from build123d import *

# Parameters (mm, degrees)
F2_R     = 0.99999
F3_R     = 2.75
F4_DEPTH = 7.5
F5_R     = 1.75
F6_DEPTH = 9.5
F7_SIZE  = 0.5


# Not quite as in the source:
# - a fillet or chamfer is up to 0.001 mm smaller than in the source, because OpenCascade refuses the exact size


with BuildPart() as f1:
    # F0 (on Front) → F1 (revolve)
    with BuildSketch(Plane.XZ):
        Polygon((0, 4), (0, 0), (17, 0), (17, 3.5), (12, 3.5), (6, 5), (6, 4), align=None)
    revolve(axis=Axis((8.5, 0, 0), (-1, 0, 0)))

    # F2 (radius 1 in the source; OpenCascade refuses exactly that, so slightly less here)
    f2_edges = [f1.edges().sort_by_distance(p)[0] for p in [
        (6, 0, -4),
    ]]
    fillet(f2_edges, radius=F2_R)

    # F3 (on face) → F4 (cut)
    with BuildSketch(Plane.YZ.offset(17)):
        Circle(F3_R)
    extrude(amount=-F4_DEPTH, mode=Mode.SUBTRACT)

    # F5 (on face) → F6 (cut, through all)
    with BuildSketch(Plane(origin=(0, 0, 0), x_dir=(0, -1, 0), z_dir=(-1, 0, 0))):
        Circle(F5_R)
    extrude(amount=-F6_DEPTH, mode=Mode.SUBTRACT)

    # F7
    f7_edges = [f1.edges().sort_by_distance(p)[0] for p in [
        (0, 0, -4),
        (0, 1.75, 0),
    ]]
    chamfer(f7_edges, length=F7_SIZE)


solid = f1.part
Verification items for the finished model (mm, model axes). A direction names the side the tool comes from. Give positions to 0.01 mm unless a question says otherwise; leave off trailing zeros. Loops run counter-clockwise (first coordinate to the right, second up) from the corner with the lowest first, then second, coordinate; pieces in that order, holes last. Notation, with made-up numbers: (-19.5, -31.5) - (34.5, -31.5) arc R8 cw to (34.5, -19.5) - close; hole circle Ø9 at (1, 20). An arc over 180 degrees is marked (long way). Write item = value, one per line. Start each with the question number.
Q1. Tool access check on faces 4 (the face through (4.937, -1.617, -0.67)), 5 (the face through (9.5, 2, 0)), 6 (the face through (2.719, -3.905, -0.867)). Record the directions out of +Z, -Z, +X, -X, +Y, -Y that give a thin tool (end or side, any length) a straight path to the whole face; none if there is none.
Q2. Cross-section at C-C, the plane x = 2. Enter the section's corners in (y, z), and give its area (3 significant figures).
Q3. Cross-section at D-D, the plane x = 7.5. Enter the section's corners in (y, z) (3 decimals).
Q4. Mould release check, pull along Z, two halves, no side actions. Record for faces 1 (the face through (0, -0.7, 2.3)), 2 (the face through (10.291, -3.834, -0.851)), 3 (the face through (13.302, -0.596, -2.685)): released by +Z, released by -Z, zero draft, split by the parting line, or undercut.
Q5. Thickness scan on line 1 (X direction, y = -2.25, z = 1); line 2 (Y direction, x = 11.5, z = -0.75); line 3 (Y direction, x = 2.5, z = 1.25). Record the ranges inside material, lowest first.
Q6. Depth check by flat-ended pin: P1, Ø5, axis at x = 13.5, z = -2.5, coming from the +Y side; P2, Ø1, axis at x = 15, y = -0.5, coming from the -Z side; P3, Ø1.5, axis at x = 15, y = 1.5, coming from the +Z side. Enter the tip coordinate at first touch or a pass-through.
Answer key:
q1.face_4 = +X, -X
q1.face_5 = +X
q1.face_6 = -X
q2.outline = circle Ø8 at (0, 0); hole circle Ø3.5 at (0, 0)
q2.area = 40.6 mm^2
q3.outline = circle Ø9.25 at (0, 0); hole circle Ø3.5 at (0, 0)
q4.face_1 = zero draft
q4.face_2 = split by the parting line
q4.face_3 = undercut
q5.line_1 = 0 to 9.5
q5.line_2 = -3.55 to -2.65, 2.65 to 3.55
q5.line_3 = -3.8 to -1.22, 1.22 to 3.8
q6.P1 = 3.5
q6.P2 = -3.5
q6.P3 = 3.42
